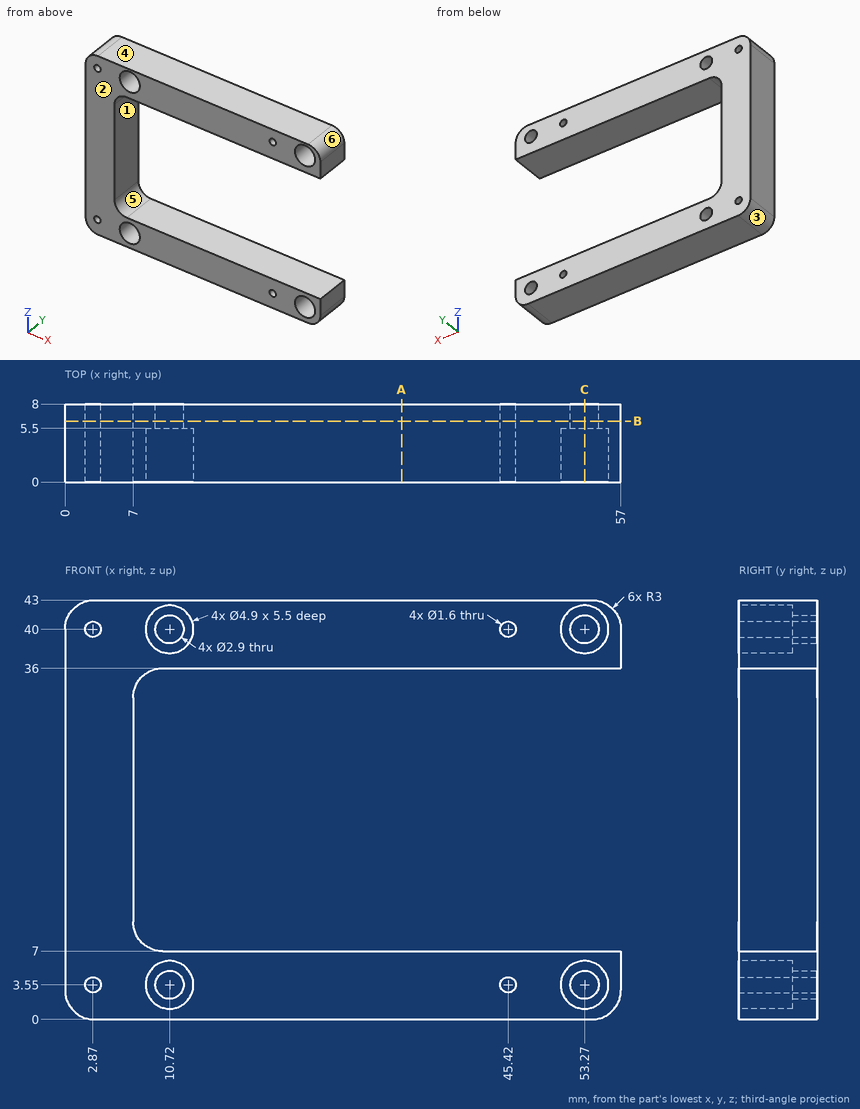
Drawing for the job (mm, zero at the part's lowest x, y, z). A direction names the side the tool comes from. Round coordinates to 2 decimals unless told otherwise and drop trailing zeros. Loops run counter-clockwise (first coordinate to the right, second up) from the corner with the lowest first, then second, coordinate; pieces in that order, holes last. Notation, with made-up numbers: (-40, 84) -> (9, 84) arc R14 ccw to (9, 101) -> close; hole circle Ø5 at (59.25, 48). An arc over 180 degrees is marked (long way). Answer in a Markdown table with one row per item.
Item 1: Saw through at B-B (y = 6.25). State how many separate pieces and enclosed holes the cut face has, and give its area (3 significant figures).
Answers below:
| item | result |
|---|---|
| separate pieces | 1 |
| enclosed holes | 8 |
| area | 963 mm² |
Item 2: Saw through at C-C (x = 53.27). Write the cut outline in (y, z), and give its area (3 significant figures).
Answers below:
| item | result |
|---|---|
| outline | (0, 0) -> (8, 0) -> (8, 2.1) -> (5.5, 2.1) -> (5.5, 1.1) -> (0, 1.1) -> close; (0, 6) -> (5.5, 6) -> (5.5, 5) -> (8, 5) -> (8, 7) -> (0, 7) -> close; (0, 36) -> (8, 36) -> (8, 38.55) -> (5.5, 38.55) -> (5.5, 37.55) -> (0, 37.55) -> close; (0, 42.45) -> (5.5, 42.45) -> (5.5, 41.45) -> (8, 41.45) -> (8, 43) -> (0, 43) -> close |
| area | 43.6 mm² |
Item 3: Mould opens along Z. For the marked faces 1, 2, 3 and 4 say: +Z half, -Z half, draft (parallel to the pull), parting line (faces both ways), or undercut.
Answers below:
| item | result |
|---|---|
| face 1 | undercut |
| face 2 | draft |
| face 3 | -Z half |
| face 4 | +Z half |
Item 4: Pin check, flat tips, straight feed: pin 1 (4 mm diameter, centred on x = 52, z = 4.5, fed in from -Y); pin 2 (1 mm diameter, centred on y = 1.5, z = 19.5, fed in from +X); pin 3 (4 mm diameter, centred on x = 10.72, z = 40, fed in from -Y). Stop position of each tip, or through.
Answers below:
| item | result |
|---|---|
| pin 1 | stops at y = 0 |
| pin 2 | stops at x = 7 |
| pin 3 | stops at y = 5.5 |
Item 5: Saw through at A-A (x = 34.5). Write the cut outline in (y, z), and give its area (3 significant figures).
Answers below:
| item | result |
|---|---|
| outline | (0, 0) -> (8, 0) -> (8, 7) -> (0, 7) -> close; (0, 36) -> (8, 36) -> (8, 43) -> (0, 43) -> close |
| area | 112 mm² |
Item 6: Drill centre lines: L1, parallel to X at y = 2.5, z = 40; L2, parallel to Z at x = 53.27, y = 6.95; L3, parallel to Z at x = 45.42, y = 6.5. Where is each one in solid material? Low to high. Write a range as [from, to].
Answers below:
| item | result |
|---|---|
| L1 | x = [0, 2.07], [3.67, 8.27], [13.17, 44.62], [46.22, 50.82], [55.72, 57] |
| L2 | z = [0, 2.1], [5, 7], [36, 38.55], [41.45, 43] |
| L3 | z = [0, 2.75], [4.35, 7], [36, 39.2], [40.8, 43] |
Item 7: Which spindle directions (+Z, -Z, +X, -X, +Y, -Y) get a long thin tool onto all of the face, cutting with end or side? Do the marked faces 5 and 6. Say none if no direction does.
Answers below:
| item | result |
|---|---|
| face 5 | +X, +Y, -Y |
| face 6 | +Z, +X, +Y, -Y |
